Can you work these out from the model? Positions are in its coordinate system, mm. A direction names the side the tool comes from. Coordinates: 2 decimals unless noted, no trailing zeros.
```python
from build123d import *

# Parameters (mm, degrees)
BOSS_EXTRUDE2_DEPTH = 15
CUT_EXTRUDE1_DEPTH  = 1


# Read off the part's stored shape, not the designer's step: Cut-Revolve-Thin2
with BuildPart() as part:
    # Sketch2 → Boss-Extrude2 (new body)
    with BuildSketch(Plane(origin=(0, 0, 0), x_dir=(1, 0, 0), z_dir=(0, 1, 0))):
        with BuildLine():
            ThreePointArc((-7.860899149, 15.635097204), (-0.183301368, -17.499039991), (8.1866917, 15.466999677))
            add(Edge.make_bspline(
                [(-7.860899149, 15.635097204), (-0.059171416, -5.64885573), (8.1866917, 15.466999677)],
                knots=[0, 0, 0, 1, 1, 1], degree=2))
        make_face()
    extrude(amount=BOSS_EXTRUDE2_DEPTH)

    # Cut-Revolve-Thin2 outline → Cut-Revolve-Thin2 (revolve, cut)
    with BuildSketch(Plane.XY):
        Polygon((17.5, 15), (10.561985935, 15), (17.5, 0.715896694), align=None)
    revolve(axis=Axis((0, 0, 0), (0, 1, 0)), mode=Mode.SUBTRACT)

    # Sketch8 → Cut-Extrude1 (cut)
    # profile 1 of 2: a face of its own
    with BuildSketch(Plane(origin=(0, 15, 0), x_dir=(1, 0, 0), z_dir=(0, 1, 0))):
        Polygon((-6.00797666, 1.283695301), (-6.00797666, -5.177491307), (-2, -5.177491307), (-2, -4.335596537), (-5.00797666, -1.946898003), (-2, 0.441800531), (-2, 1.283695301), align=None)
        Polygon((-3.50398833, -4.493701766), (-5.00797666, -4.493701766), (-5.00797666, -3.2993525), align=None, mode=Mode.SUBTRACT)
        Polygon((-5.00797666, 0.283695301), (-3.50398833, 0.283695301), (-5.00797666, -0.910653966), align=None, mode=Mode.SUBTRACT)
    # profile 2 of 2: a face of its own
    with BuildSketch(Plane(origin=(0, 15, 0), x_dir=(1, 0, 0), z_dir=(0, 1, 0))):
        Polygon((2, 1.283695301), (3, 1.283695301), (3, -1.216304699), (6, -1.216304699), (6, 1.283695301), (7, 1.283695301), (7, -5.493701766), (6, -5.493701766), (6, -2.216304699), (2, -2.216304699), align=None)
    extrude(amount=-CUT_EXTRUDE1_DEPTH, mode=Mode.SUBTRACT)


solid = part.part
```
Item 1: We'd pull the mould along X, two halves only. Please class faces 3 (the face through (-0.562, 12.519, 11.753)), 4 (the face through (-4, 14.5, -1.284)), 5 (the face through (-4.6, 15, 4.2)): +X half, -X half, draft (parallel to the pull), parting line (faces both ways), or undercut.
Results are:
face 3: parting line
face 4: undercut
face 5: draft
Item 2: I need wall thicknesses on line 1 along Y through (x, z) = (15, 7.5); line 2 along X through (y, z) = (9.75, -7); line 3 along Y through (x, z) = (-8, -8). Which ranges of each line are inside material? Lowest first, please.
Results are:
line 1: y = 0 to 2.22
line 2: x = -11.09 to -3.42, 3.63 to 11.09
line 3: y = 0 to 13.45
Item 3: I'm going to push flat-ended pins straight in: P1, Ø1.1, axis at y = 14.5, z = 3, coming from the +X side; P2, Ø1.1, axis at y = 14.5, z = 1, coming from the +X side; P3, Ø0.8, axis at x = -4.5, y = 14.5, coming from the -Z side. Where does each tip first touch, or does it pass through?
Results are:
P1: stops at x = 10.69
P2: stops at x = 11.03
P3: stops at z = -9.11
Item 4: On a 3-axis mill with a long thin cutter (end or side, diameter ignored), from which of +Z, -Z, +X, -X, +Y, -Y can I reach the whole of each face in a straight line? I mean faces 1 (the face through (-4.4, 15, 0.2)), 2 (the face through (7, 14.5, 2.1)). Say none if no direction works.
Results are:
face 1: +Z, -Z, +X, -X, +Y
face 2: +Y
